The listing builds one solid part. Answer for the finished solid, in the listing's coordinates (mm). A direction names the side the tool comes from. Coordinates: 2 decimals unless noted, no trailing zeros. Write each loop counter-clockwise with the first axis right and the second up, starting at its lowest first coordinate (ties: lowest second). Pieces come first, ordered by that corner, then holes. Notation, with made-up numbers: M -10.75,13.5 L 4.25,13.5 A29 ccw 4.25,42.5 Z; hole C 77.5,40.25 d1. An arc over 180 degrees is marked long. Answer as CSV lines item,"result". Start each with the question number.
```python
from build123d import *

# Parameters (mm, degrees)
F0_W     = 60
F0_H     = 30
F1_DEPTH = 90
F2_R     = 2.5
F3_DEPTH = 40
F4_R     = 1.25
F5_DEPTH = 40


with BuildPart() as f1:
    # F0 (on Top) → F1 (new body)
    with BuildSketch(Plane.XY):
        Rectangle(F0_W, F0_H)
    extrude(amount=F1_DEPTH)

    # F2 (on face) → F3 (cut)
    with BuildSketch(Plane(origin=(0, 0, 0), x_dir=(1, 0, 0), z_dir=(0, 0, -1))):
        Circle(F2_R)
    extrude(amount=-F3_DEPTH, mode=Mode.SUBTRACT)

    # F4 (on face) → F5 (cut)
    with BuildSketch(Plane.XY.offset(90)):
        with Locations((-15, 0)):
            Circle(F4_R)
        with Locations((15, 0)):
            Circle(F4_R)
    extrude(amount=-F5_DEPTH, mode=Mode.SUBTRACT)


solid = f1.part
```
1) For a pull along X with two mould halves and no side action, classify faces 4 (the face through (0, -15, 44)), 5 (the face through (-30, 0, 44)), 6 (the face through (15, 0, 50)) as +X half, -X half, draft (parallel to the pull), parting line (faces both ways), or undercut.
2) Each of these flat-tipped pins is pushed along its axis until it touches: P1, Ø3, axis at x = 0, y = 0, coming from the -Z side; P2, Ø2, axis at x = -15, y = 0, coming from the +Z side. Where does it stop, or does it pass through?
3) Which of the six approach directions +Z, -Z, +X, -X, +Y, -Y give full straight-line access (tool end or side, diameter ignored) to faces 1 (the face through (-16.25, 0.05, 70.28)), 2 (the face through (0, 0, 40)), 3 (the face through (0, 0, 90))?
4) The part is cut by section B-B (x = 15). Determine the outline of the cut face in (y, z).
5) The part is cut by section C-C (x = 0). Determine the outline of the cut face in (y, z), then the cut area to 3 significant figures.
6) Find the intervals of material crossed by line 1 (Y direction, x = 15, z = 64.5); line 2 (Y direction, x = 0, z = 18); line 3 (Z direction, x = 0, y = 0.25), in increasing order. Write a range as from..to.
7) The part is cut by section A-A (y = 0). Determine the outline of the cut face in (x, z).
Completed:
1,face 4,"draft"
1,face 5,"-X half"
1,face 6,"undercut"
2,P1,"z = 40"
2,P2,"z = 50"
3,face 1,"+Z"
3,face 2,"-Z"
3,face 3,"+Z, +X, -X, +Y, -Y"
4,outline,"M -15,0 L 15,0 L 15,90 L 1.25,90 L 1.25,50 L -1.25,50 L -1.25,90 L -15,90 Z"
5,outline,"M -15,0 L -2.5,0 L -2.5,40 L 2.5,40 L 2.5,0 L 15,0 L 15,90 L -15,90 Z"
5,area,"2,500 mm²"
6,line 1,"-15..-1.25, 1.25..15"
6,line 2,"-15..-2.5, 2.5..15"
6,line 3,"40..90"
7,outline,"M -30,0 L -2.5,0 L -2.5,40 L 2.5,40 L 2.5,0 L 30,0 L 30,90 L 16.25,90 L 16.25,50 L 13.75,50 L 13.75,90 L -13.75,90 L -13.75,50 L -16.25,50 L -16.25,90 L -30,90 Z"
